Job drawing, mm, ordinate dimensions from the low corner. One solid piece. Give positions to 0.01 mm unless a question says otherwise; leave off trailing zeros. Order: outer loops, then holes, each group sorted by start corner. A loop starts at its lowest first (then second) coordinate and runs counter-clockwise, first axis right, second up. Notation, with made-up numbers: (-39, 12.25) - (-12, 12.25) arc R28 ccw to (-12, 40.25) - close; hole circle Ø1 at (-20, -16.75). An arc over 180 degrees is marked (long way). Use a Markdown table: item, result. Add a question column.
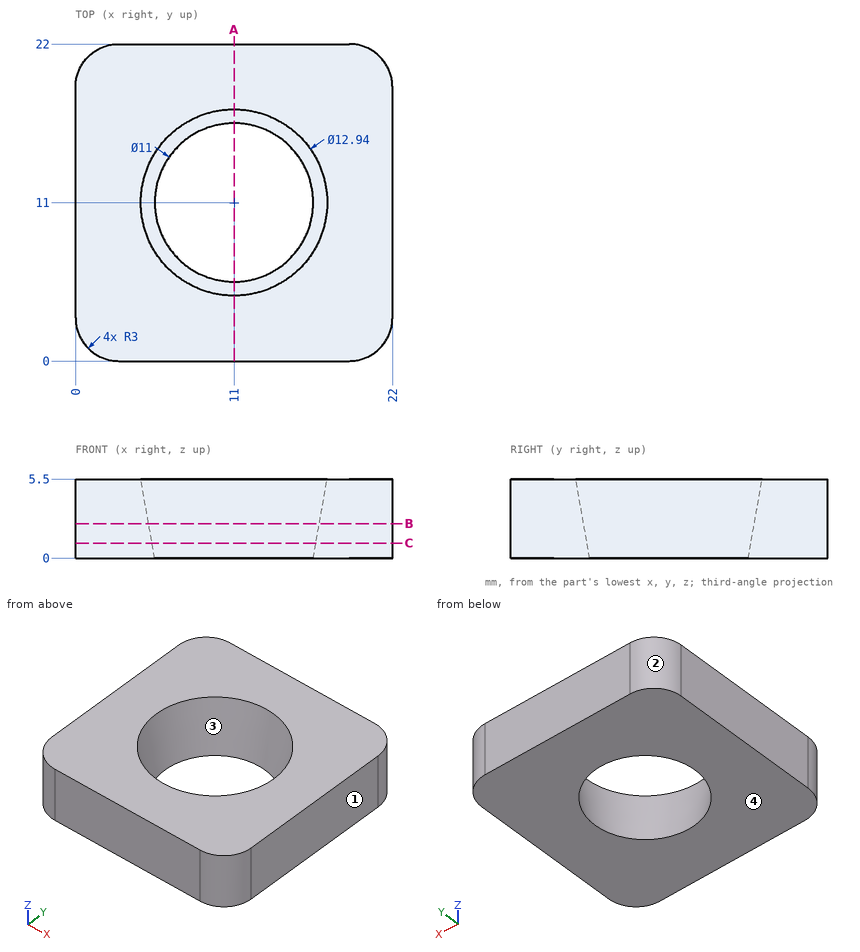
1. Cut at A-A (x = 11). Write the cut outline in (y, z).
2. Mould opens along X. For the marked faces 1, 2, 3 and 4 say: released by +X, released by -X, zero draft, split by the parting line, or undercut.
3. Pin check, flat tip, straight feed: P1, Ø2, axis at y = 5.5, z = 1.5, coming from the -X side. Stop position of the tip, or through.
4. Cut at B-B (z = 2.4). Write the cut outline in (x, y).
5. Cut at C-C (z = 1.05). Write the cut outline in (x, y) (1 decimal).
6. Drill centre lines: probe 1 along X at (y, z) = (5.25, 5.25) (1 decimal); probe 2 along Y at (x, z) = (16.5, 3.4) (1 decimal); probe 3 along X at (y, z) = (15, 4.9). Where is each one in solid material? Low to high. Write a range as [from, to].
Responses:
| question | item | result |
|---|---|---|
| 1 | outline | (0, 0) - (5.5, 0) - (4.53, 5.5) - (0, 5.5) - close; (16.5, 0) - (22, 0) - (22, 5.5) - (17.47, 5.5) - close |
| 2 | face 1 | released by +X |
| 2 | face 2 | released by -X |
| 2 | face 3 | undercut |
| 2 | face 4 | zero draft |
| 3 | P1 | stops at x = 0 |
| 4 | outline | (0, 3) arc R3 ccw to (3, 0) - (19, 0) arc R3 ccw to (22, 3) - (22, 19) arc R3 ccw to (19, 22) - (3, 22) arc R3 ccw to (0, 19) - close; hole circle Ø11.85 at (11, 11) |
| 5 | outline | (0, 3) arc R3 ccw to (3, 0) - (19, 0) arc R3 ccw to (22, 3) - (22, 19) arc R3 ccw to (19, 22) - (3, 22) arc R3 ccw to (0, 19) - close; hole circle Ø11.4 at (11, 11) |
| 6 | probe 1 | x = [0, 8.1], [13.9, 22] |
| 6 | probe 2 | y = [0, 8.4], [13.6, 22] |
| 6 | probe 3 | x = [0, 6.05], [15.95, 22] |
